For this review, use the dimensioned drawing (mm, ordinates from the lowest corner) and the shaded views. A direction names the side the tool comes from. Give positions to 0.01 mm unless a question says otherwise; leave off trailing zeros. Write each loop counter-clockwise with the first axis right and the second up, starting at its lowest first coordinate (ties: lowest second). Pieces come first, ordered by that corner, then holes. Notation, with made-up numbers: (-32, 63.25) -> (-12, 63.25) arc R33 cw to (-12, 101.25) -> close; hole circle Ø2 at (79, 30). An arc over 180 degrees is marked (long way). Write each question's results on one line, items separated by ' | '. Start each with the question number.
(1) Take a section at C-C (y = 4.25). State the section outline as (x, z) points.
(2) Take a section at A-A (z = 14). State the section outline as (x, y) points, plus the area to 4 significant figures.
(3) Take a section at D-D (z = 10). State the section outline as (x, y) points, plus the area to 3 significant figures.
(4) Mouldability with a two-part tool opening along X and no side actions: class the marked faces 4, 5 and 6 as released by +X, released by -X, zero draft, split by the parting line, or undercut.
(5) Take a section at B-B (x = 27). State the section outline as (y, z) points, plus the area to 3 significant figures.
(6) Clearance check with flat-ended pins moving along their axes: pin 1 (10 mm diameter, centred on x = 22, z = 11.5, fed in from +Y); pin 2 (10 mm diameter, centred on x = 24.5, y = 15.5, fed in from -Z); pin 3 (1.5 mm diameter, centred on x = 29, y = 8, fed in from -Z). State where each tip first meets the part, or that it passes through.
(7) For the marked faces 1, 2 and 3, list the 3-axis set-ups (+Z, -Z, +X, -X, +Y, -Y) from which the entire face can be reached by the end or side of a thin tool; tool diameter is ignored.
(8) To check wall thickness, follow probe 1 along X at (y, z) = (19.5, 14); probe 2 along X at (y, z) = (18.9, 14); probe 3 along Z at (x, y) = (6, 20.05). State the ranges of each line that lie inside material, in increasing order.
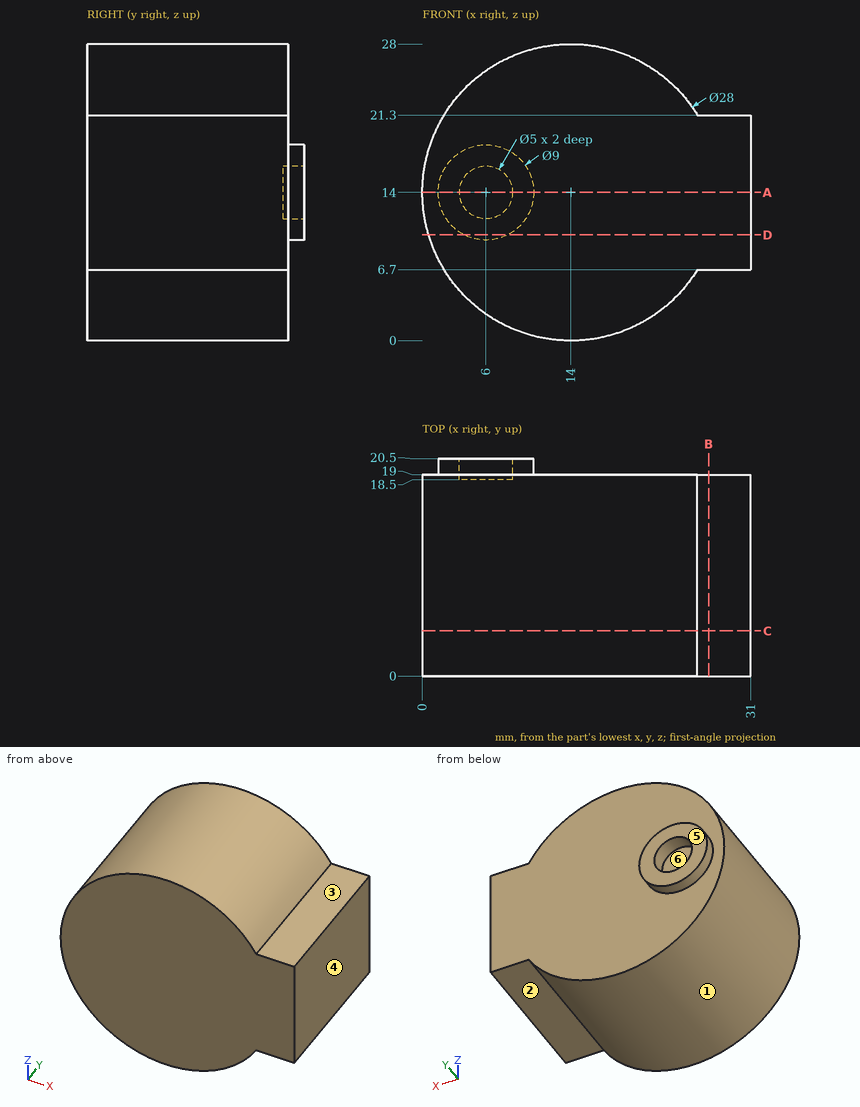
Report:
1) outline: (25.95, 6.7) -> (31, 6.7) -> (31, 21.3) -> (25.95, 21.3) arc R14 ccw (long way) to start
2) outline: (0, 0) -> (31, 0) -> (31, 19) -> (10.5, 19) -> (10.5, 20.5) -> (8.5, 20.5) -> (8.5, 18.5) -> (3.5, 18.5) -> (3.5, 20.5) -> (1.5, 20.5) -> (1.5, 19) -> (0, 19) -> close | area: 592.5 mm2
3) outline: (0.58, 0) -> (31, 0) -> (31, 19) -> (8.06, 19) -> (8.06, 20.5) -> (3.94, 20.5) -> (3.94, 19) -> (0.58, 19) -> close | area: 584 mm2
4) face 4: released by +X | face 5: zero draft | face 6: undercut
5) outline: (0, 6.7) -> (19, 6.7) -> (19, 21.3) -> (0, 21.3) -> close | area: 277 mm2
6) pin 1: y = 19 | pin 2: z = 1.13 | pin 3: z = 6.7
7) face 1: +Y, -Y | face 2: -Z, +X, +Y, -Y | face 3: +Z, +X, +Y, -Y
8) probe 1: 1.5 to 3.5, 8.5 to 10.5 | probe 2: 0 to 3.5, 8.5 to 31 | probe 3: 9.5 to 11.5, 16.5 to 18.5
